Can you work these out from the model? Positions are in its coordinate system, mm. A direction names the side the tool comes from. Round coordinates to 2 decimals unless told otherwise and drop trailing zeros. Loops run counter-clockwise (first coordinate to the right, second up) from the corner with the lowest first, then second, coordinate; pieces in that order, holes last. Notation, with made-up numbers: (16.5, 56.25) -> (65.5, 56.25) arc R18 ccw to (65.5, 71.25) -> close; hole circle Ø1 at (85, -1). An arc over 180 degrees is marked (long way). Write each question's results on one line, items separated by ' | '.
from build123d import *

# Parameters (mm, degrees)
ESQUISSE1_R                  = 0.550000000000003
ESQUISSE1_R_2                = 1.050000000000001
BOSS_EXTRU_1_DEPTH           = 5
BOSS_EXTRU_2_DEPTH           = 10
ENL_V_MAT_EXTRU_1_DEPTH      = 61.96067460568836
ENL_V_MAT_EXTRU_1_DEPTH_BACK = 61.96067460568836
CONG_1_R                     = 4
ESQUISSE4_R                  = 1.0999999999999948
ENL_V_MAT_EXTRU_2_DEPTH      = 81.96368978508603


with BuildPart() as part:
    # Esquisse1 → Boss.-Extru.1 (new body)
    with BuildSketch(Plane(origin=(0, 0, 0), x_dir=(0, 0, -1), z_dir=(1, 0, 0))):
        with BuildLine():
            ThreePointArc((-48.767999999999994, 0), (-39.18749628154784, 29.028571428571436), (-14.210176870748295, 46.65178128755695))
            ThreePointArc((-14.210176870748295, 46.65178128755695), (-11.168776456672475, 52.35758986489808), (-16.874585034013602, 55.39899027897389))
            ThreePointArc((-16.874585034013602, 55.39899027897389), (-46.53515183433805, 34.47142857142858), (-57.91199999999999, 0))
            ThreePointArc((-57.91199999999999, 0), (-53.339999999999996, -4.571999999999996), (-48.767999999999994, 0))
        make_face()
        with Locations((-53.339999999999996, 0)):
            Circle(ESQUISSE1_R, mode=Mode.SUBTRACT)
        with Locations((-15.542380952380952, 51.02538578326543)):
            Circle(ESQUISSE1_R_2, mode=Mode.SUBTRACT)
    extrude(amount=BOSS_EXTRU_1_DEPTH)

    # Esquisse2 → Boss.-Extru.2 (add)
    with BuildSketch(Plane(origin=(5, 0, 0), x_dir=(0, 0, -1), z_dir=(1, 0, 0))):
        with BuildLine():
            Line((-31.772627007894677, 48.41797101301542), (-26.755896427700776, 40.77302822148666))
            ThreePointArc((-26.755896427700776, 40.77302822148666), (-20.692866519079303, 44.16019813388031), (-14.210176870748292, 46.65178128755695))
            ThreePointArc((-14.210176870748292, 46.65178128755695), (-11.168776456672475, 52.35758986489808), (-16.874585034013602, 55.3989902789739))
            ThreePointArc((-16.874585034013602, 55.3989902789739), (-24.57277899140668, 52.44023528398287), (-31.772627007894677, 48.41797101301542))
        make_face()
    extrude(amount=BOSS_EXTRU_2_DEPTH)

    # Esquisse3 → Enlèv. mat.-Extru.1 (cut, two sides: drawn at the far end of the back side and taken through both)
    with BuildSketch(Plane(origin=(-2.205e-14, 48.41797101301542, 31.77262700789469), x_dir=(-1, 0, -6.9e-16), z_dir=(0, 0.836061110184684, 0.5486363276677492)).offset(-ENL_V_MAT_EXTRU_1_DEPTH_BACK)):
        Polygon((-4.500000000000018, -21.069257970907522), (-10.500000000000023, -21.069257970907522), (-10.500000000000023, -5.000000000000025), (-4.500000000000011, -5.0000000000000195), align=None)
    extrude(amount=ENL_V_MAT_EXTRU_1_DEPTH + ENL_V_MAT_EXTRU_1_DEPTH_BACK, mode=Mode.SUBTRACT)

    # Congé1
    cong_1_edges = [part.edges().sort_by_distance(p)[0] for p in [
        (5, 44.595499617251036, 29.264261717797726),
        (15, 44.595499617251036, 29.264261717797726),
    ]]
    fillet(cong_1_edges, radius=CONG_1_R)

    # Esquisse4 → Enlèv. mat.-Extru.2 (cut, through all)
    with BuildSketch(Plane.ZY.offset(-10.500000000000023)):
        with Locations((15.542380952380947, 51.02538578326543)):
            Circle(ESQUISSE4_R)
    extrude(amount=-ENL_V_MAT_EXTRU_2_DEPTH, mode=Mode.SUBTRACT)


solid = part.part
1. If we section it at B-B (x = 11.75): List the corners of the cut face in (y, z) for me.
Final values:
outline: (40.81, 26.7) arc R48.77 cw to (46.65, 14.21) arc R4.57 ccw to (55.4, 16.87) arc R57.91 ccw to (48.46, 31.71) -> close; hole circle Ø2.2 at (51.03, 15.54)
2. If we section it at A-A (x = 2.5): List the corners of the cut face in (y, z) for me, then the cut area to 3 significant figures.
Final values:
outline: (0, 48.77) arc R48.77 cw to (46.65, 14.21) arc R4.57 ccw to (55.4, 16.87) arc R57.91 ccw to (0, 57.91) arc R4.57 ccw to start; hole circle Ø1.1 at (0, 53.34); hole circle Ø2.1 at (51.03, 15.54) | area: 683 mm2
3. If we section it at C-C (z = 50): List the corners of the cut face in (x, y) for me, then the cut area to 3 significant figures.
Final values:
outline: (0, -3.12) -> (5, -3.12) -> (5, 29.22) -> (0, 29.22) -> close | area: 162 mm2
4. Will these pins go through, and if not, where does the flat tip stop? pin 1 (5 mm diameter, centred on x = 6.5, z = 34, fed in from +Y); pin 2 (4 mm diameter, centred on x = 5, y = 48.5, fed in from -Z); pin 3 (1 mm diameter, centred on x = 11.5, y = 44.5, fed in from +Z).
Final values:
pin 1: y = 48.6 | pin 2: z = 11.01 | pin 3: z = 29.5
5. If we section it at D-D (y = 25): List the corners of the cut face in (x, z) for me, then the cut area to 3 significant figures.
Final values:
outline: (0, 41.87) -> (5, 41.87) -> (5, 52.24) -> (0, 52.24) -> close | area: 51.8 mm2
6. On a 3-axis mill with a long thin cutter (end or side, diameter ignored), from which of +Z, -Z, +X, -X, +Y, -Y can I reach the whole of each face in a straight line? I mean faces 4 (the face through (7.54, 47.09, 24.92)), 5 (the face through (9.99, 44.65, 29.3)), 6 (the face through (4.06, 33.96, 35)). Say none if no direction works.
Final values:
face 4: -Z, +Y | face 5: +Z, +X, -Y | face 6: -Z, +X, -X, -Y
7. Please list where these lines run through material, in increasing order: line 1 (X direction, y = 21, z = 45.5); line 2 (Y direction, x = 3.75, z = 53.34); line 3 (Z direction, x = 7, y = 48). Write a range as from..to.
Final values:
line 1: 0..5 | line 2: -4.57..-0.55, 0.55..22.55 | line 3: 25.52..32.14
8. We'd pull the mould along Z, two halves only. Please class faces 1 (the face through (5, 21, 47)), 2 (the face through (6.2, 43.85, 30.14)), 3 (the face through (12.72, 50.05, 16.05)): pulls with the +Z half, pulls with the -Z half, needs draft (parallel to the pull), parting line crosses it, or undercut.
Final values:
face 1: needs draft | face 2: pulls with the +Z half | face 3: undercut
